```python
from build123d import *

# Parameters (mm, degrees)
SKETCH_1_R      = 1.5
SKETCH_1_R_2    = 2.5
EXTRUDE_2_DEPTH = 5


with BuildPart() as part:
    # 草圖1 → 填料-伸長2 (new body)
    with BuildSketch(Plane.XY):
        with BuildLine():
            Line((-20, 30), (-20, -30))
            Line((-20, -30), (17.897858345, -30))
            ThreePointArc((17.897858345, -30), (37.816442632, -18.5), (37.816442632, 4.5))
            Line((37.816442632, 4.5), (17.320508076, 40))
            ThreePointArc((17.320508076, 40), (-5.176380902, 49.318516526), (-20, 30))
        make_face()
        with Locations((-12, -8)):
            Circle(SKETCH_1_R, mode=Mode.SUBTRACT)
        with Locations((-12, -22)):
            Circle(SKETCH_1_R, mode=Mode.SUBTRACT)
        with Locations((12, -22)):
            Circle(SKETCH_1_R, mode=Mode.SUBTRACT)
        with Locations((12, -8)):
            Circle(SKETCH_1_R, mode=Mode.SUBTRACT)
        with Locations((0, 35)):
            Circle(SKETCH_1_R_2, mode=Mode.SUBTRACT)
        with Locations((30, -16.961524227)):
            Circle(SKETCH_1_R_2, mode=Mode.SUBTRACT)
    extrude(amount=EXTRUDE_2_DEPTH)


solid = part.part
```
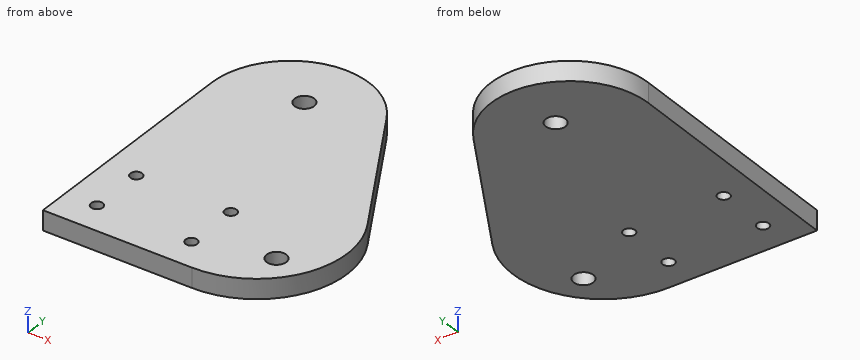
Verification items for the finished model (mm, model axes). Give positions to 0.01 mm unless a question says otherwise; leave off trailing zeros. Write each loop counter-clockwise with the first axis right and the second up, starting at its lowest first coordinate (ties: lowest second). Pieces come first, ordered by that corner, then holes. Notation, with made-up numbers: M 24,85.5 L 61,85.5 A30 cw 61,122.5 Z; hole C 72,29 d4. An arc over 180 degrees is marked long. One line per question, with ' | ' between items.
1) Thickness scan on line 1 along Y through (x, z) = (12, 2.2); line 2 along Y through (x, z) = (12.5, 2.55); line 3 along Y through (x, z) = (32, 3.85). Record the ranges inside material, lowest first. Write a range as [from, to].
Result:
line 1: y = [-30, -23.5], [-20.5, -9.5], [-6.5, 46] | line 2: y = [-30, -23.41], [-20.59, -9.41], [-6.59, 45.61] | line 3: y = [-25.17, -18.46], [-15.46, 14.57]
2) Section check B-B on x = 12. Enter the section's corners in (y, z).
Result:
outline: M -30,0 L -23.5,0 L -23.5,5 L -30,5 Z; M -20.5,0 L -9.5,0 L -9.5,5 L -20.5,5 Z; M -6.5,0 L 46,0 L 46,5 L -6.5,5 Z
3) Section check A-A on x = 0. Enter the section's corners in (y, z).
Result:
outline: M -30,0 L 32.5,0 L 32.5,5 L -30,5 Z; M 37.5,0 L 50,0 L 50,5 L 37.5,5 Z
4) Gauge pin test, flat ends, axial feed: pin 1 Ø3 at (x, y) = (0, 35) entering from +Z; pin 2 Ø1 at (y, z) = (13.5, 1) entering from +X; pin 3 Ø1 at (y, z) = (-1.5, 2) entering from +X; pin 4 Ø1 at (x, z) = (22, 1) entering from +Y. Record the tip position at first contact, or that the pin passes through.
Result:
pin 1: passes through | pin 2: stops at x = 32.91 | pin 3: stops at x = 40.35 | pin 4: stops at y = 32.76
5) Section check C-C on y = -22. Enter the section's corners in (x, z).
Result:
outline: M -20,0 L -13.5,0 L -13.5,5 L -20,5 Z; M -10.5,0 L 10.5,0 L 10.5,5 L -10.5,5 Z; M 13.5,0 L 35.33,0 L 35.33,5 L 13.5,5 Z
6) Section check D-D on z = 3.25. Enter the section's corners in (x, y).
Result:
outline: M -20,-30 L 17.9,-30 A23 ccw 37.82,4.5 L 17.32,40 A20 ccw -20,30 Z; hole C -12,-22 d3; hole C -12,-8 d3; hole C 0,35 d5; hole C 12,-22 d3; hole C 12,-8 d3; hole C 30,-16.96 d5
